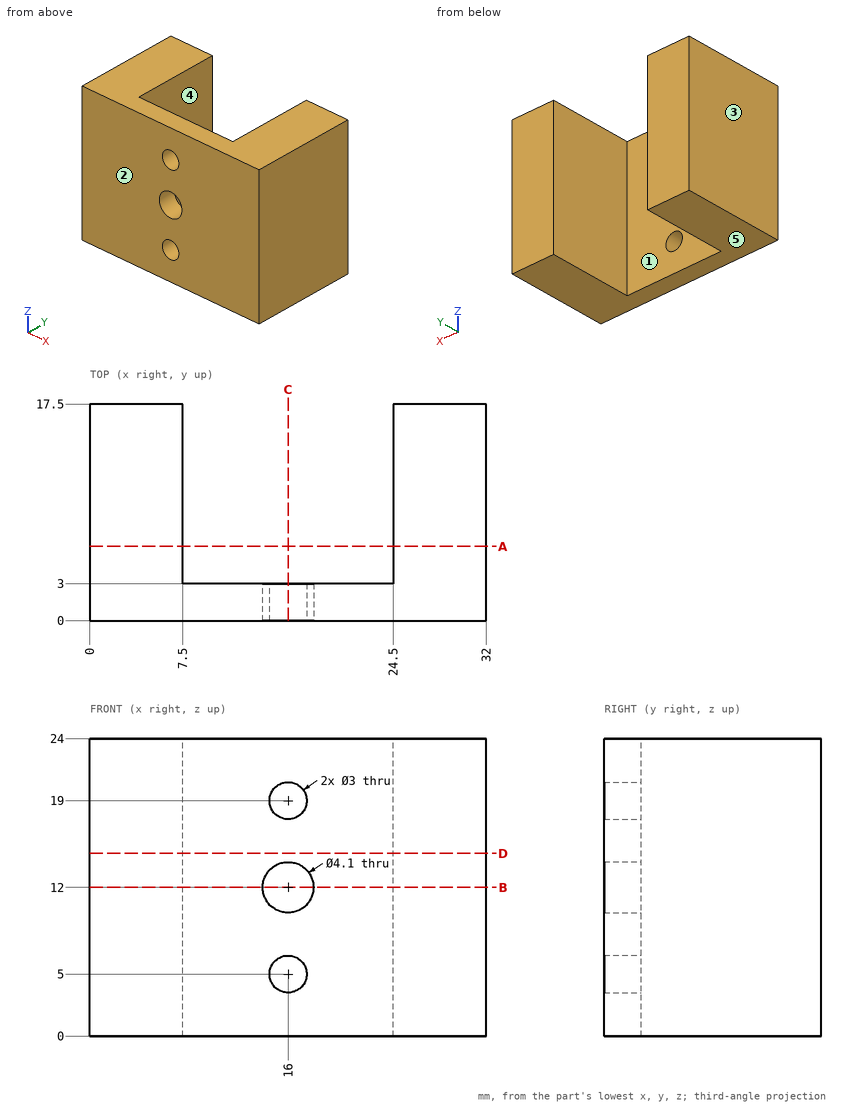
Geometry: see drawing. Coordinates: mm, zero at the bounding-box minimum. A direction names the side the tool comes from. Give positions to 0.01 mm unless a question says otherwise; leave off trailing zeros. Loops run counter-clockwise (first coordinate to the right, second up) from the corner with the lowest first, then second, coordinate; pieces in that order, holes last. Notation, with made-up numbers: (70, 50) -> (106, 50) arc R7 cw to (106, 56) -> close; hole circle Ø3 at (-0.75, -16). An arc over 180 degrees is marked (long way). Answer as a JSON object with one key per item and string values. Group by question number.
Item 1: Pull-direction query (X, two-part tool) for the marked faces 1, 2 and 3; classes: released by +X, released by -X, zero draft, split by the parting line, or undercut.
Item 2: Cut plane A-A, the plane y = 6. Return the cut outline in (x, z), and give its area (3 significant figures).
Item 3: Cut plane C-C, the plane x = 16. Return the cut outline in (y, z), and give its area (3 significant figures).
Item 4: Pin query (flat end, axial travel): P1, Ø2.5, axis at x = 16, z = 5, coming from the -Y side; P2, Ø5, axis at x = 14.5, z = 15, coming from the +Y side. Return the tip coordinate at first contact, or that it passes through.
Item 5: Line query: probe 1 along Z at (x, y) = (16, 1.4); probe 2 along X at (y, z) = (5.25, 20.5); probe 3 along X at (y, z) = (2.35, 5). Output: solid intervals per line, ascending.
Item 6: Cut plane D-D, the plane z = 14.75. Return the cut outline in (x, y), and give its area (4 significant figures).
Item 7: Reachability of the marked faces 4 and 5 from +Z, -Z, +X, -X, +Y, -Y: full face, straight path, thin tool, end or side. Return the list, or none.
Item 8: Cut plane B-B, the plane z = 12. Return the cut outline in (x, y), and give its area (3 significant figures).
Checks:
{
 "1": {"face 1": "undercut", "face 2": "zero draft", "face 3": "released by -X"},
 "2": {"outline": "(0, 0) -> (7.5, 0) -> (7.5, 24) -> (0, 24) -> close; (24.5, 0) -> (32, 0) -> (32, 24) -> (24.5, 24) -> close", "area": "360 mm²"},
 "3": {"outline": "(0, 0) -> (3, 0) -> (3, 3.5) -> (0, 3.5) -> close; (0, 6.5) -> (3, 6.5) -> (3, 9.95) -> (0, 9.95) -> close; (0, 14.05) -> (3, 14.05) -> (3, 17.5) -> (0, 17.5) -> close; (0, 20.5) -> (3, 20.5) -> (3, 24) -> (0, 24) -> close", "area": "41.7 mm²"},
 "4": {"P1": "passes through", "P2": "stops at y = 3"},
 "5": {"probe 1": "z = 0 to 3.5, 6.5 to 9.95, 14.05 to 17.5, 20.5 to 24", "probe 2": "x = 0 to 7.5, 24.5 to 32", "probe 3": "x = 0 to 14.5, 17.5 to 32"},
 "6": {"outline": "(0, 0) -> (32, 0) -> (32, 17.5) -> (24.5, 17.5) -> (24.5, 3) -> (7.5, 3) -> (7.5, 17.5) -> (0, 17.5) -> close", "area": "313.5 mm²"},
 "7": {"face 4": "+Z, -Z, +Y", "face 5": "-Z, +X, -X, +Y, -Y"},
 "8": {"outline": "(0, 0) -> (13.95, 0) -> (13.95, 3) -> (7.5, 3) -> (7.5, 17.5) -> (0, 17.5) -> close; (18.05, 0) -> (32, 0) -> (32, 17.5) -> (24.5, 17.5) -> (24.5, 3) -> (18.05, 3) -> close", "area": "301 mm²"}
}
